CAD build for the part. Positions are in the model's coordinates, mm. Face numbers are marked on the shaded views. A direction names the side the tool comes from. Coordinates: 2 decimals unless noted, no trailing zeros. Write each loop counter-clockwise with the first axis right and the second up, starting at its lowest first coordinate (ties: lowest second). Pieces come first, ordered by that corner, then holes. Notation, with made-up numbers: (63, 9) - (71, 9) arc R20 cw to (71, 19) - close; hole circle Ø7 at (27, 87). An arc over 180 degrees is marked (long way). Answer in a Markdown table with one row per item. Add a question column.
Q1. Band-saw the part on D-D (z = 0). List the corners of the cut face in (x, y) (3 decimals).
Q2. Band-saw the part on C-C (x = 12). List the corners of the cut face in (y, z), and give its area (3 significant figures).
Q3. Band-saw the part on B-B (z = -20). List the corners of the cut face in (x, y), and give its area (3 significant figures).
Q4. Drill centre lines: line 1 along Z through (x, y) = (-12, 2); line 2 along X through (y, z) = (1.9, -21); line 3 along X through (y, z) = (2.25, -6.5) (3 decimals). Where is each one in solid material? Low to high. Write a range as from..to.
Q5. Two-plate mould, pull along X, no slides. Class the marked faces 1, 2 and 3: +X half, -X half, draft (parallel to the pull), parting line (faces both ways), or undercut.
Q6. Pin check, flat tips, straight feed: pin 1 (5.5 mm diameter, centred on x = 0, z = -21, fed in from -Y); pin 2 (2.5 mm diameter, centred on x = -12.5, y = 1.5, fed in from +Z); pin 3 (8 mm diameter, centred on x = 15, z = -1.5, fed in from +Y); pin 4 (10 mm diameter, centred on x = 8, z = -13, fed in from +Y). Stop position of each tip, or through.
Q7. Band-saw the part on A-A (x = 0). List the corners of the cut face in (y, z), and give its area (3 significant figures).
Q8. 3-axis set-ups, long thin cutter, end or side, ignore diameter. For the marked faces 4, 5, 6, 7 and 8: which of +Z, -Z, +X, -X, +Y, -Y reach the whole face in a straight line?
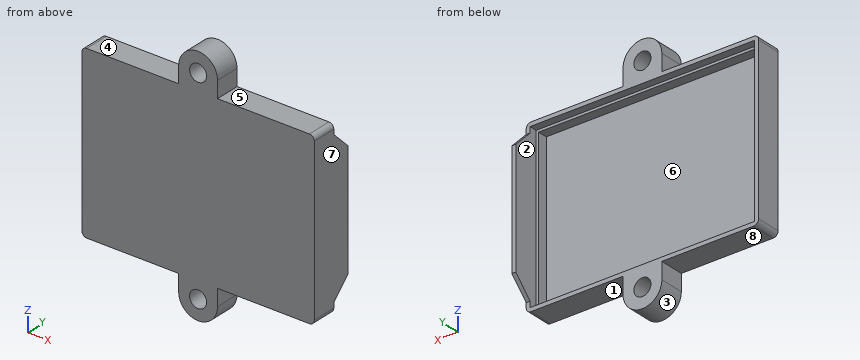
```python
from build123d import *

# Parameters (mm, degrees)
SKETCH1_W           = 47.85
SKETCH1_H           = 35.2
BOSS_EXTRUDE1_DEPTH = 5.1
SKETCH2_W           = 46.25
SKETCH2_H           = 33.6
CUT_EXTRUDE1_DEPTH  = 1.6
SKETCH3_W           = 45.25
SKETCH3_H           = 32.6
CUT_EXTRUDE2_DEPTH  = 2
BOSS_EXTRUDE2_DEPTH = 0.8
FILLET1_R           = 1
SKETCH6_R           = 1.75
BOSS_EXTRUDE3_DEPTH = 5.1


with BuildPart() as part:
    # Sketch1 → Boss-Extrude1 (new body)
    with BuildSketch(Plane(origin=(0, 0, 0), x_dir=(1, 0, 0), z_dir=(0, 1, 0))):
        Rectangle(SKETCH1_W, SKETCH1_H)
    extrude(amount=BOSS_EXTRUDE1_DEPTH)

    # Sketch2 → Cut-Extrude1 (cut)
    with BuildSketch(Plane(origin=(0, 5.1, 0), x_dir=(1, 0, 0), z_dir=(0, 1, 0))):
        Rectangle(SKETCH2_W, SKETCH2_H)
    extrude(amount=-CUT_EXTRUDE1_DEPTH, mode=Mode.SUBTRACT)

    # Sketch3 → Cut-Extrude2 (cut)
    with BuildSketch(Plane(origin=(0, 3.5, 0), x_dir=(1, 0, 0), z_dir=(0, 1, 0))):
        Rectangle(SKETCH3_W, SKETCH3_H)
    extrude(amount=-CUT_EXTRUDE2_DEPTH, mode=Mode.SUBTRACT)

    # Sketch4 → Boss-Extrude2 (add)
    with BuildSketch(Plane(origin=(23.925, 0, 0), x_dir=(0, 0, -1), z_dir=(1, 0, 0))):
        Polygon((-15.6, 5.1), (-11.85, 8.85), (11.85, 8.85), (15.6, 5.1), align=None)
    extrude(amount=-BOSS_EXTRUDE2_DEPTH)

    # Fillet1
    fillet1_edges = [part.edges().sort_by_distance(p)[0] for p in [
        (-23.925, 2.55, -17.6),
        (23.925, 2.55, -17.6),
        (23.925, 2.55, 17.6),
        (-23.925, 2.55, 17.6),
    ]]
    fillet(fillet1_edges, radius=FILLET1_R)

    # Sketch6 → Boss-Extrude3 (add)
    # profile 1 of 2: a face of its own
    with BuildSketch(Plane.XZ):
        with BuildLine():
            Line((-4, 17.6), (4, 17.6))
            Line((4, 17.6), (4, 21))
            ThreePointArc((4, 21), (0, 25), (-4, 21))
            Line((-4, 21), (-4, 17.6))
        make_face()
        with Locations(Location((0, 21, 0), (0, 0, 270))):
            Circle(SKETCH6_R, mode=Mode.SUBTRACT)
    # profile 2 of 2: a face of its own
    with BuildSketch(Plane.XZ):
        with BuildLine():
            Line((-4, -17.6), (-4, -21))
            ThreePointArc((-4, -21), (0, -25), (4, -21))
            Line((4, -21), (4, -17.6))
            Line((4, -17.6), (-4, -17.6))
        make_face()
        with Locations(Location((0, -21, 0), (0, 0, 270))):
            Circle(SKETCH6_R, mode=Mode.SUBTRACT)
    extrude(amount=-BOSS_EXTRUDE3_DEPTH)


solid = part.part
```
Checked values:
| question | item | result |
|---|---|---|
| 1 | outline | (-23.925, 0) - (23.925, 0) - (23.925, 8.85) - (23.125, 8.85) - (23.125, 3.5) - (22.625, 3.5) - (22.625, 1.5) - (-22.625, 1.5) - (-22.625, 3.5) - (-23.125, 3.5) - (-23.125, 5.1) - (-23.925, 5.1) - close |
| 2 | outline | (0, -17.6) - (5.1, -17.6) - (5.1, -16.8) - (3.5, -16.8) - (3.5, -16.3) - (1.5, -16.3) - (1.5, 16.3) - (3.5, 16.3) - (3.5, 16.8) - (5.1, 16.8) - (5.1, 17.6) - (0, 17.6) - close |
| 2 | area | 60.6 mm² |
| 3 | outline | (-4, 0) - (-1.44, 0) - (-1.44, 5.1) - (-4, 5.1) - close; (1.44, 0) - (4, 0) - (4, 5.1) - (1.44, 5.1) - close |
| 3 | area | 26.2 mm² |
| 4 | line 1 | z = -17.6..-16.3, 16.3..17.6 |
| 4 | line 2 | x = -4..-1.75, 1.75..4 |
| 4 | line 3 | x = -23.925..-22.625, 22.625..23.925 |
| 5 | face 1 | draft |
| 5 | face 2 | undercut |
| 5 | face 3 | parting line |
| 6 | pin 1 | stops at y = 0 |
| 6 | pin 2 | stops at z = 17.6 |
| 6 | pin 3 | stops at y = 1.5 |
| 6 | pin 4 | stops at y = 5.1 |
| 7 | outline | (0, -25) - (5.1, -25) - (5.1, -22.75) - (0, -22.75) - close; (0, -19.25) - (5.1, -19.25) - (5.1, -16.8) - (3.5, -16.8) - (3.5, -16.3) - (1.5, -16.3) - (1.5, 16.3) - (3.5, 16.3) - (3.5, 16.8) - (5.1, 16.8) - (5.1, 19.25) - (0, 19.25) - close; (0, 22.75) - (5.1, 22.75) - (5.1, 25) - (0, 25) - close |
| 7 | area | 100 mm² |
| 8 | face 4 | +Z, -X, +Y, -Y |
| 8 | face 5 | +Z, +X, +Y, -Y |
| 8 | face 6 | +Y |
| 8 | face 7 | +Z, -Z, +X, +Y, -Y |
| 8 | face 8 | -Z, -X, +Y, -Y |
